Check sheet for the modelled part. Datum: model origin and axes. Units: mm. Round coordinates to 2 decimals unless told otherwise and drop trailing zeros. Loops run counter-clockwise (first coordinate to the right, second up) from the corner with the lowest first, then second, coordinate; pieces in that order, holes last. Notation, with made-up numbers: M -37.5,23 L -15.5,23 A16 ccw -15.5,50 Z; hole C 63,89 d8. An arc over 180 degrees is marked long. Write item = value, one per line. Start each with the question number.
(1) Go/stop test with flat-tipped pins: P1, Ø1.5, axis at y = -1.5, z = 7.5, coming from the +X side; P2, Ø1.7, axis at x = -0.29, y = -7.93, coming from the +Z side; P3, Ø3, axis at y = -5, z = 2, coming from the -X side. Record where each tip stops, or that it passes through.
(2) Cross-section at A-A on x = 2.5. Record the boundary of the cut face in (y, z).
(3) Cross-section at D-D on z = 5.75. State how many separate pieces and enclosed holes the cut face has, plus the area to 3 significant figures.
(4) Cross-section at B-B on y = -2. Record the boundary of the cut face in (x, z), plus the area to 3 significant figures.
(5) Scan lines: L1, parallel to Y at x = 0, z = 8.25 (3 decimals); L2, parallel to X at y = 5.5, z = 1.5; L3, parallel to Z at x = -10.5, y = 2.75. Record each from-to range of solid material in increasing order. Write a range as from..to.
(6) Mould release check, pull along Y, two halves, no side actions. Record for faces 1 (the face through (3, 6, 6.35)), 2 (the face through (-1.38, -6.2, 9.57)), 3 (the face through (5.34, 5.83, 3.22)): pulls with the +Y half, pulls with the -Y half, needs draft (parallel to the pull), parting line crosses it, or undercut.
(7) Cross-section at C-C on z = 9. Record the boundary of the cut face in (x, y) (3 decimals), plus the area to 3 significant figures.
from build123d import *

# Parameters (mm, degrees)
SKETCH1_R           = 12.7
BOSS_EXTRUDE1_DEPTH = 12.7
SKETCH2_R           = 3.175
CUT_EXTRUDE1_DEPTH  = 22.997045256
SKETCH3_R           = 15.493591624
SKETCH3_R_2         = 6.35
CUT_EXTRUDE2_DEPTH  = 6.35
SKETCH4_R           = 0.635
CUT_EXTRUDE3_DEPTH  = 20.05


with BuildPart() as part:
    # Sketch1 → Boss-Extrude1 (new body)
    with BuildSketch(Plane.XY):
        Circle(SKETCH1_R)
    extrude(amount=BOSS_EXTRUDE1_DEPTH)

    # Sketch2 → Cut-Extrude1 (cut, through all)
    with BuildSketch(Plane.XY.offset(12.7)):
        Circle(SKETCH2_R)
    extrude(amount=-CUT_EXTRUDE1_DEPTH, mode=Mode.SUBTRACT)

    # Sketch3 → Cut-Extrude2 (cut)
    with BuildSketch(Plane.XY.offset(12.7)):
        Circle(SKETCH3_R)
        Circle(SKETCH3_R_2, mode=Mode.SUBTRACT)
    extrude(amount=-CUT_EXTRUDE2_DEPTH, mode=Mode.SUBTRACT)

    # Sketch4 → Cut-Extrude3 (cut, through all)
    with BuildSketch(Plane.XY.offset(6.35)):
        with Locations((0.288137957, 7.93226845)):
            Circle(SKETCH4_R)
        with Locations((5.812705114, 5.405216508)):
            Circle(SKETCH4_R)
        with Locations((7.93226845, -0.288137957)):
            Circle(SKETCH4_R)
        with Locations((5.405216508, -5.812705114)):
            Circle(SKETCH4_R)
        with Locations((-0.288137957, -7.93226845)):
            Circle(SKETCH4_R)
        with Locations((-5.812705114, -5.405216508)):
            Circle(SKETCH4_R)
        with Locations((-7.93226845, 0.288137957)):
            Circle(SKETCH4_R)
        with Locations((-5.405216508, 5.812705114)):
            Circle(SKETCH4_R)
    extrude(amount=-CUT_EXTRUDE3_DEPTH, mode=Mode.SUBTRACT)


solid = part.part
Result:
q1.P1 = 6.31
q1.P2 = 6.35
q1.P3 = -12.21
q2.outline = M -12.45,0 L -1.96,0 L -1.96,12.7 L -5.84,12.7 L -5.84,6.35 L -12.45,6.35 Z; M 1.96,0 L 12.45,0 L 12.45,6.35 L 5.84,6.35 L 5.84,12.7 L 1.96,12.7 Z
q3.separate_pieces = 1
q3.enclosed_holes = 9
q3.area = 465 mm^2
q4.outline = M -12.54,0 L -2.47,0 L -2.47,12.7 L -6.03,12.7 L -6.03,6.35 L -12.54,6.35 Z; M 2.47,0 L 12.54,0 L 12.54,6.35 L 6.03,6.35 L 6.03,12.7 L 2.47,12.7 Z
q4.area = 173 mm^2
q5.L1 = -6.35..-3.175, 3.175..6.35
q5.L2 = -11.45..-5.96, -4.85..5.18, 6.44..11.45
q5.L3 = 0..6.35
q6.face_1 = needs draft
q6.face_2 = parting line crosses it
q6.face_3 = undercut
q7.outline = C 0,0 d12.7; hole C 0,0 d6.35
q7.area = 95.0 mm^2
